Geometry: see drawing. Coordinates: mm, zero at the bounding-box minimum. A direction names the side the tool comes from. Give positions to 0.01 mm unless a question says otherwise; leave off trailing zeros. Write each loop counter-clockwise with the first axis right and the second up, starting at its lowest first coordinate (ties: lowest second). Pieces come first, ordered by that corner, then holes. Notation, with made-up numbers: (-32.5, 78.5) -> (11.5, 78.5) arc R13 cw to (11.5, 92.5) -> close; hole circle Ø10 at (-23.5, 68). An arc over 180 degrees is marked (long way). Use CSV: the item, a comma, the result in double quotes. Start each with the question number.
1) Section C-C (z = 8.5). Output: boundary loops of the cut face in (x, y), plus the area to 3 significant figures.
2) Section A-A (x = 2.5). Output: boundary loops of the cut face in (y, z), plus the area to 3 significant figures.
3) Set-up query: the marked faces 1, 2 and 3. Return all of +Z, -Z, +X, -X, +Y, -Y with unobstructed straight access to the full face (end or side cutting, diameter ignored); none if empty.
4) Material intervals for line 1 (Y direction, x = 1, z = 4); line 2 (Z direction, x = 2.15, y = 1.25); line 3 (Z direction, x = 4.2, y = 3.25), sorted ascending. Write a range as [from, to].
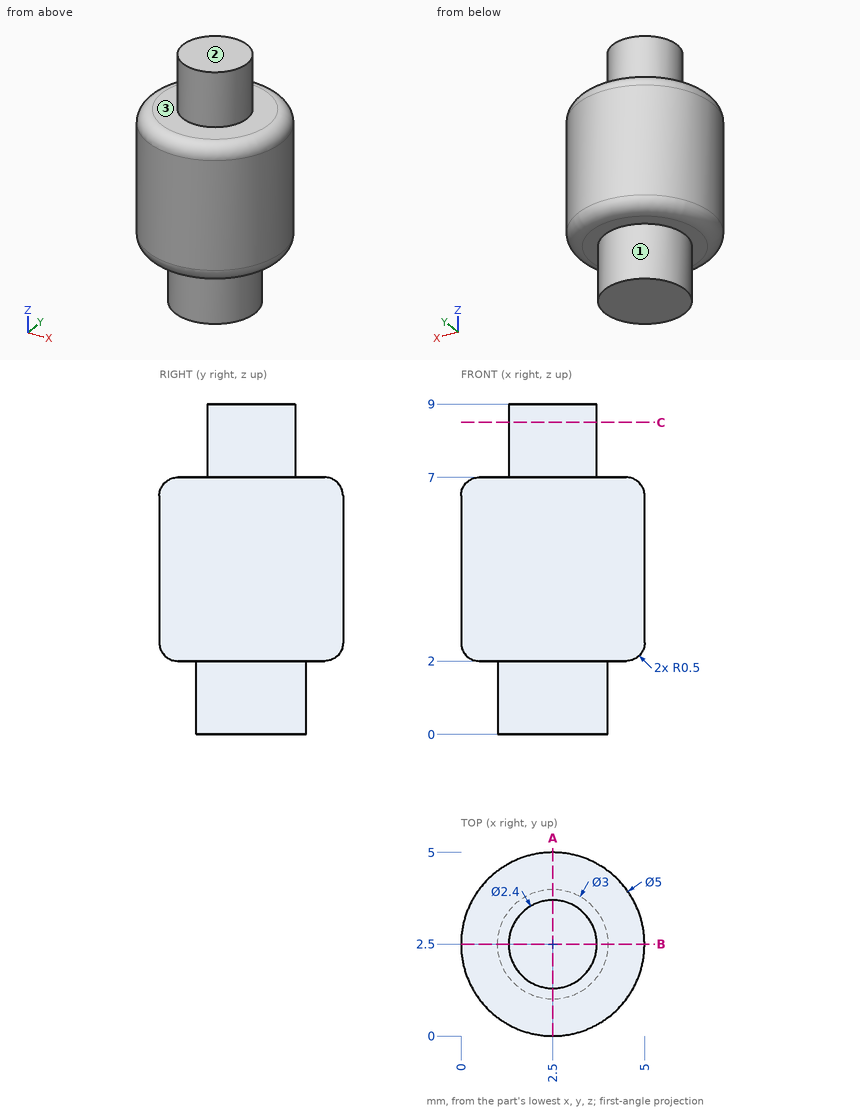
Answers follow:
1,outline,"circle Ø2.4 at (2.5, 2.5)"
1,area,"4.52 mm^2"
2,outline,"(0, 2.5) arc R0.5 ccw to (0.5, 2) -> (1, 2) -> (1, 0) -> (4, 0) -> (4, 2) -> (4.5, 2) arc R0.5 ccw to (5, 2.5) -> (5, 6.5) arc R0.5 ccw to (4.5, 7) -> (3.7, 7) -> (3.7, 9) -> (1.3, 9) -> (1.3, 7) -> (0.5, 7) arc R0.5 ccw to (0, 6.5) -> close"
2,area,"35.6 mm^2"
3,face 1,"-Z"
3,face 2,"+Z, +X, -X, +Y, -Y"
3,face 3,"+Z"
4,line 1,"y = [0.5, 4.5]"
4,line 2,"z = [0, 7]"
4,line 3,"z = [2, 7]"
